from build123d import *

# Parameters (mm, degrees)
EXTRUDE_1_DEPTH     = 22.2
EXTRUDE_2_DEPTH     = 4.5
SKETCH_3_R          = 1.5
CUT_EXTRUDE_1_DEPTH = 47.223181414
CUT_EXTRUDE_3_DEPTH = 3.7
CUT_EXTRUDE_4_REACH = 67.816
SKETCH_6_W          = 9
SKETCH_6_H          = 7.6
SKETCH_6_W_2        = 11
SKETCH_6_H_2        = 6
CUT_EXTRUDE_5_REACH = 67.816
SKETCH_7_W          = 5
SKETCH_7_H          = 5
SKETCH_8_R          = 1.5
EXTRUDE_3_DEPTH     = 0.8
SKETCH_10_W         = 60.4
SKETCH_10_H         = 26.7
CUT_EXTRUDE_7_DEPTH = 66.815575664


with BuildPart() as part:
    # 草圖1 → 填料-伸長1 (new body)
    with BuildSketch(Plane.XY):
        Polygon((-25.794213562, 27.05), (25.794213562, 27.05), (30.2, 22.644213562), (30.2, -22.644213562), (25.794213562, -27.05), (-25.794213562, -27.05), (-30.2, -22.644213562), (-30.2, 22.644213562), align=None)
        Polygon((-29.4, 22.312842712), (-25.462842712, 26.25), (25.462842712, 26.25), (29.4, 22.312842712), (29.4, -22.312842712), (25.462842712, -26.25), (-25.462842712, -26.25), (-29.4, -22.312842712), align=None, mode=Mode.SUBTRACT)
    extrude(amount=EXTRUDE_1_DEPTH)

    # 草圖2 → 填料-伸長2 (add)
    with BuildSketch(Plane(origin=(0, 0, 0), x_dir=(-1, 0, 0), z_dir=(0, 0, -1))):
        Polygon((-30.2, 22.644213562), (-25.794213562, 27.05), (25.794213562, 27.05), (30.2, 22.644213562), (30.2, -22.644213562), (25.794213562, -27.05), (-25.794213562, -27.05), (-30.2, -22.644213562), align=None)
    extrude(amount=EXTRUDE_2_DEPTH)

    # 草圖3 → 除料-伸長1 (cut, through all)
    with BuildSketch(Plane.XY):
        with Locations((25.2, 22.03)):
            Circle(SKETCH_3_R)
        with Locations(Location((25.2, -22.03, 0), (0, 0, 180))):
            Circle(SKETCH_3_R)
        with Locations((-25.2, -22.03)):
            Circle(SKETCH_3_R)
        with Locations(Location((-25.2, 22.03, 0), (0, 0, 180))):
            Circle(SKETCH_3_R)
    extrude(amount=-CUT_EXTRUDE_1_DEPTH, mode=Mode.SUBTRACT)

    # 草圖5 → 除料-伸長3 (cut)
    with BuildSketch(Plane.XY):
        with BuildLine():
            Line((-25.234050993, 18.530165643), (-25.234050993, -18.530165643))
            ThreePointArc((-25.234050993, -18.530165643), (-22.715358839, -19.564932394), (-21.700544406, -22.091729589))
            Line((-21.700544406, -22.091729589), (21.700544406, -22.091729589))
            ThreePointArc((21.700544406, -22.091729589), (22.737758998, -19.542557689), (25.297360416, -18.531354412))
            Line((25.297360416, -18.531354412), (25.297360416, 18.531354412))
            ThreePointArc((25.297360416, 18.531354412), (22.56426249, 19.727200014), (21.74608079, 22.596076045))
            Line((21.74608079, 22.596076045), (-21.74608079, 22.596076045))
            ThreePointArc((-21.74608079, 22.596076045), (-22.543539666, 19.751136578), (-25.234050993, 18.530165643))
        make_face()
    extrude(amount=-CUT_EXTRUDE_3_DEPTH, mode=Mode.SUBTRACT)

    # 草圖6 → 除料-伸長4 (cut, up to next)
    with BuildSketch(Plane.XZ.offset(27.05), mode=Mode.PRIVATE) as cut_extrude_4_sk1:
        with Locations((6.7, 4.9)):
            Rectangle(SKETCH_6_W, SKETCH_6_H)
    cut_extrude_4_tool1 = extrude(cut_extrude_4_sk1.sketch, amount=-CUT_EXTRUDE_4_REACH, mode=Mode.PRIVATE) & part.part
    # 草圖6 → 除料-伸長4 (cut, up to next)
    with BuildSketch(Plane.XZ.offset(27.05), mode=Mode.PRIVATE) as cut_extrude_4_sk2:
        with Locations((-11.7, 14.2)):
            Rectangle(SKETCH_6_W_2, SKETCH_6_H_2)
    cut_extrude_4_tool2 = extrude(cut_extrude_4_sk2.sketch, amount=-CUT_EXTRUDE_4_REACH, mode=Mode.PRIVATE) & part.part
    add(cut_extrude_4_tool1.solids().sort_by_distance((6.7, -27.05, 4.9))[0], mode=Mode.SUBTRACT)
    add(cut_extrude_4_tool2.solids().sort_by_distance((-11.7, -27.05, 14.2))[0], mode=Mode.SUBTRACT)

    # 草圖7 → 除料-伸長5 (cut, up to next)
    with BuildSketch(Plane(origin=(0, 27.05, 0), x_dir=(1, 0, 0), z_dir=(0, 1, 0)), mode=Mode.PRIVATE) as cut_extrude_5_sk1:
        with Locations((0, -8.85)):
            Rectangle(SKETCH_7_W, SKETCH_7_H)
    cut_extrude_5_tool1 = extrude(cut_extrude_5_sk1.sketch, amount=-CUT_EXTRUDE_5_REACH, mode=Mode.PRIVATE) & part.part
    add(cut_extrude_5_tool1.solids().sort_by_distance((0, 27.05, 8.85))[0], mode=Mode.SUBTRACT)

    # 草圖8 → 填料-伸長3 (add)
    with BuildSketch(Plane(origin=(0, 0, -4.5), x_dir=(-1, 0, 0), z_dir=(0, 0, -1))):
        Polygon((30.2, -22.644213562), (25.794213562, -27.05), (-25.794213562, -27.05), (-30.2, -22.644213562), (-30.2, 22.644213562), (-25.794213562, 27.05), (25.794213562, 27.05), (30.2, 22.644213562), align=None)
        with Locations(Location((25.2, -22.03, 0), (0, 0, 180))):
            Circle(SKETCH_8_R, mode=Mode.SUBTRACT)
        with Locations((-25.2, -22.03)):
            Circle(SKETCH_8_R, mode=Mode.SUBTRACT)
        with Locations(Location((-25.2, 22.03, 0), (0, 0, 180))):
            Circle(SKETCH_8_R, mode=Mode.SUBTRACT)
        with Locations((25.2, 22.03)):
            Circle(SKETCH_8_R, mode=Mode.SUBTRACT)
    extrude(amount=EXTRUDE_3_DEPTH)

    # 草圖10 → 除料-伸長7 (cut, through all)
    with BuildSketch(Plane(origin=(0, 27.05, 0), x_dir=(1, 0, 0), z_dir=(0, 1, 0))):
        with Locations((0, -8.85)):
            Rectangle(SKETCH_10_W, SKETCH_10_H)
    extrude(amount=-CUT_EXTRUDE_7_DEPTH, mode=Mode.SUBTRACT)


solid = part.part
Part model, mm, in its own coordinate system. Round coordinates to 2 decimals unless told otherwise and drop trailing zeros. Loops run counter-clockwise (first coordinate to the right, second up) from the corner with the lowest first, then second, coordinate; pieces in that order, holes last. Notation, with made-up numbers: (8.5, -39) - (48.5, -39) arc R33 cw to (48.5, 0) - close; hole circle Ø1 at (6.25, 42). An arc over 180 degrees is marked (long way). Answer as a JSON object with one key per item and string values.
Item 1: Pin check, flat tips, straight feed: pin 1 (5 mm diameter, centred on x = -25.2, y = 22.03, fed in from -Z); pin 2 (1.8 mm diameter, centred on x = 25.2, y = -22.03, fed in from -Z). Stop position of each tip, or through.
Output:
{"pin 1": "z = -5.3", "pin 2": "through"}
Item 2: Pull direction Y, two halves, no side cores. Call faces 1 (the face through (-24.875, 20.566, -4.894)), 2 (the face through (0, 0, -5.3)), 3 (the face through (-28.028, -24.816, -4.894)): pulls with the +Y half, pulls with the -Y half, needs draft (parallel to the pull), parting line crosses it, or undercut.
Output:
{"face 1": "undercut", "face 2": "needs draft", "face 3": "pulls with the -Y half"}
Item 3: Band-saw the part on A-A on z = -4.75. List the corners of the cut face in (x, y).
Output:
{"outline": "(-30.2, -22.64) - (-25.79, -27.05) - (25.79, -27.05) - (30.2, -22.64) - (30.2, 22.64) - (25.79, 27.05) - (-25.79, 27.05) - (-30.2, 22.64) - close; hole circle Ø3 at (-25.2, -22.03); hole circle Ø3 at (-25.2, 22.03); hole circle Ø3 at (25.2, -22.03); hole circle Ø3 at (25.2, 22.03)"}
Item 4: Wall check: L1, parallel to X at y = 22.03, z = -4.85; L2, parallel to Y at x = 25.2, z = -5.05; L3, parallel to Y at x = -26, z = -4.7. Give the ranges that are in metal, low to high.
Output:
{"L1": "-30.2 to -26.7, -23.7 to 23.7, 26.7 to 30.2", "L2": "-27.05 to -23.53, -20.53 to 20.53, 23.53 to 27.05", "L3": "-26.84 to -23.3, -20.76 to 20.76, 23.3 to 26.84"}
